Can you work these out from the drawing? Everything is in mm from the part's minimum corner. Round coordinates to 2 decimals unless told otherwise and drop trailing zeros. Order: outer loops, then holes, each group sorted by start corner. A loop starts at its lowest first (then second) coordinate and runs counter-clockwise, first axis right, second up. Notation, with made-up numbers: M 18.25,-27.5 L 27.25,-27.5 A20 cw 27.25,-12.5 Z; hole C 42,1.5 d3. An arc over 180 degrees is marked long. Use one line per item in the form item = value. Start each with the question number.
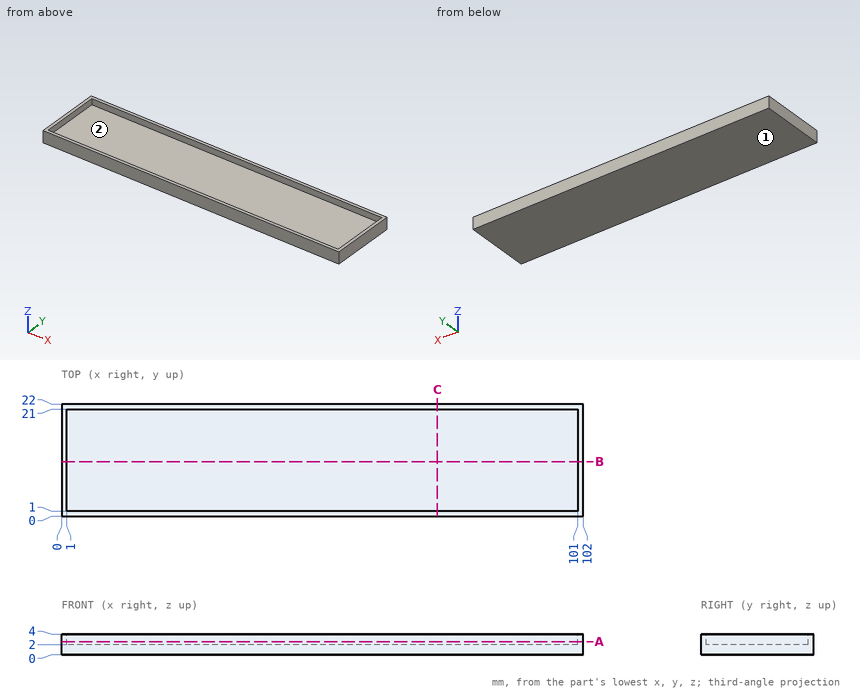
1) If we mould it in two halves opening along Y, with no side actions, what happens to the marked faces 1 and 2? For each: +Y half, -Y half, draft (parallel to the pull), parting line (faces both ways), or undercut.
2) If I drill on line 1 (Y direction, x = 5.5, z = 3.4); line 2 (X direction, y = 17, z = 2.3); line 3 (Z direction, x = 91, y = 8.75), over which ranges is the centre line in solid material (lowest first)?
3) If we section it at A-A on z = 2.6: Write out the boundary of the cut face in (x, y), then the cut area to 3 significant figures.
4) Will these pins go through, and if not, where does the flat tip stop? pin 1 Ø5 at (x, y) = (21.5, 10.5) entering from +Z; pin 2 Ø1.6 at (x, z) = (74.5, 2.5) entering from -Y.
5) If we section it at C-C on x = 73.5: Write out the boundary of the cut face in (y, z), then the cut area to 3 significant figures.
6) If we section it at B-B on y = 10.75: Write out the boundary of the cut face in (x, z), then the cut area to 3 significant figures.
Completed:
q1.face_1 = draft
q1.face_2 = undercut
q2.line_1 = 0 to 1, 21 to 22
q2.line_2 = 0 to 1, 101 to 102
q2.line_3 = 0 to 2
q3.outline = M 0,0 L 102,0 L 102,22 L 0,22 Z; hole M 1,1 L 101,1 L 101,21 L 1,21 Z
q3.area = 244 mm²
q4.pin_1 = 2
q4.pin_2 = 0
q5.outline = M 0,0 L 22,0 L 22,4 L 21,4 L 21,2 L 1,2 L 1,4 L 0,4 Z
q5.area = 48.0 mm²
q6.outline = M 0,0 L 102,0 L 102,4 L 101,4 L 101,2 L 1,2 L 1,4 L 0,4 Z
q6.area = 208 mm²
